Read the model definition and answer for the solid it produces. Units are mm, in the model's axes. A direction names the side the tool comes from. Round coordinates to 2 decimals unless told otherwise and drop trailing zeros. Order: outer loops, then holes, each group sorted by start corner. A loop starts at its lowest first (then second) coordinate and runs counter-clockwise, first axis right, second up. Notation, with made-up numbers: M 5.25,53.5 L 43.25,53.5 A27 ccw 43.25,78.5 Z; hole C -22,-1 d11. An arc over 180 degrees is marked long. Use one line per item in the form item = value. Start each with the question number.
from build123d import *

# Parameters (mm, degrees)
SKETCH1_W           = 38.5
SKETCH1_H           = 88.5
BOSS_EXTRUDE1_DEPTH = 28
SKETCH2_W           = 34.5
SKETCH2_H           = 24
CUT_EXTRUDE1_DEPTH  = 88.5
FILLET1_R           = 2
FILLET2_R           = 2
FILLET3_R           = 2
FILLET4_R           = 2
FILLET5_R           = 2
SKETCH3_W           = 84.5
SKETCH3_H           = 2
CUT_EXTRUDE2_DEPTH  = 2


with BuildPart() as part:
    # Sketch1 → Boss-Extrude1 (new body)
    with BuildSketch(Plane(origin=(0, 0, 0), x_dir=(0, 1, 0), z_dir=(0, 0, 1))):
        Rectangle(SKETCH1_W, SKETCH1_H)
    extrude(amount=BOSS_EXTRUDE1_DEPTH)

    # Sketch2 → Cut-Extrude1 (cut)
    with BuildSketch(Plane.YZ.offset(44.25)):
        with Locations((-2, 16)):
            Rectangle(SKETCH2_W, SKETCH2_H)
    extrude(amount=-CUT_EXTRUDE1_DEPTH, mode=Mode.SUBTRACT)

    # Fillet1
    fillet1_edges = [part.edges().sort_by_distance(p)[0] for p in [
        (0, 15.25, 4),
    ]]
    fillet(fillet1_edges, radius=FILLET1_R)

    # Fillet2
    fillet2_edges = [part.edges().sort_by_distance(p)[0] for p in [
        (0, 15.25, 28),
    ]]
    fillet(fillet2_edges, radius=FILLET2_R)

    # Fillet3
    fillet3_edges = [part.edges().sort_by_distance(p)[0] for p in [
        (0, -19.25, 4),
    ]]
    fillet(fillet3_edges, radius=FILLET3_R)

    # Fillet4
    fillet4_edges = [part.edges().sort_by_distance(p)[0] for p in [
        (44.25, 15.25, 16),
        (44.25, 14.664213562, 4.585786438),
        (44.25, 18.25, 28),
        (44.25, 15.835786438, 27.414213562),
        (44.25, -2, 4),
        (44.25, -19.25, 1),
        (44.25, -18.664213562, 3.414213562),
    ]]
    fillet(fillet4_edges, radius=FILLET4_R)

    # Fillet5
    fillet5_edges = [part.edges().sort_by_distance(p)[0] for p in [
        (-44.25, 15.25, 16),
        (-44.25, 14.664213562, 4.585786438),
        (-44.25, 15.835786438, 27.414213562),
        (-44.25, -2, 4),
        (-44.25, -19.25, 1),
        (-44.25, -18.664213562, 3.414213562),
        (-44.25, 18.25, 28),
    ]]
    fillet(fillet5_edges, radius=FILLET5_R)

    # Sketch3 → Cut-Extrude2 (cut)
    with BuildSketch(Plane(origin=(0, 19.25, 0), x_dir=(-1, 0, 0), z_dir=(0, 1, 0))):
        with Locations((0, 25)):
            Rectangle(SKETCH3_W, SKETCH3_H)
    extrude(amount=-CUT_EXTRUDE2_DEPTH, mode=Mode.SUBTRACT)


solid = part.part
Item 1: For a pull along Z with two mould halves and no side action, classify faces 6 (the cylindrical face through (43.65, -18.68, 1.01)), 7 (the cylindrical face through (-43.68, -1.79, 3.4)), 8 (the flat face through (-42.25, 18, 25)), 9 (the flat face through (42.25, 18, 25)) as pulls with the +Z half, pulls with the -Z half, needs draft (parallel to the pull), parting line crosses it, or undercut.
Item 2: Section A-A (x = 24) is taken. Write down the section's boundary in (y, z), and give its area (3 significant figures).
Item 3: Find the intervals of material crossed by L1, parallel to Z at x = -38, y = 17.5; L2, parallel to Y at x = -23.5, z = 17.75; L3, parallel to Y at x = 28, z = 24.25, in increasing order. Write a range as [from, to].
Item 4: Given P1, Ø1, axis at x = 9, y = 18, coming from the -Z side; P2, Ø1, axis at x = -23, y = 4.5, coming from the +Z side, each flat-ended and moving along its own axis, determine where each tip first touches the part or whether it passes through.
Item 5: A tool of negligible diameter and unlimited length cuts with its end or side. For faces 1 (the flat face through (1, 18, 26)), 2 (the flat face through (1, -2, 4)), 3 (the cylindrical face through (-43.68, 15.85, 16.14)), 4 (the flat face through (-1, 0, 0)), 5 (the cylindrical face through (43.65, 15.82, 16.14)), from which of +Z, -Z, +X, -X, +Y, -Y can it reach the whole face along a straight path? Write none if from no direction.
Item 6: Section B-B (z = 9.75) is taken. Write down the section's boundary in (x, y).
Item 7: Section C-C (y = 5) is taken. Write down the section's boundary in (x, z), and give its area (3 significant figures).
The answers:
q1.face_6 = needs draft
q1.face_7 = pulls with the +Z half
q1.face_8 = undercut
q1.face_9 = undercut
q2.outline = M -19.25,0 L 19.25,0 L 19.25,24 L 17.25,24 L 17.25,26 L 19.25,26 L 19.25,28 L 17.25,28 A2 ccw 15.25,26 L 15.25,6 A2 cw 13.25,4 L -17.25,4 A2 ccw -19.25,2 Z
q2.area = 245 mm²
q3.L1 = [0, 24], [26, 28]
q3.L2 = [15.25, 19.25]
q3.L3 = [15.25, 17.25]
q4.P1 = 0
q4.P2 = 4
q5.face_1 = +Y
q5.face_2 = +Z, +X, -X, -Y
q5.face_3 = +Z, -X, -Y
q5.face_4 = -Z, +X, -X, +Y, -Y
q5.face_5 = +Z, +X, -Y
q6.outline = M -44.25,17.25 A2 ccw -42.25,15.25 L 42.25,15.25 A2 ccw 44.25,17.25 L 44.25,19.25 L -44.25,19.25 Z
q7.outline = M -44.25,0 L 44.25,0 L 44.25,2 A2 ccw 42.25,4 L -42.25,4 A2 ccw -44.25,2 Z
q7.area = 352 mm²
